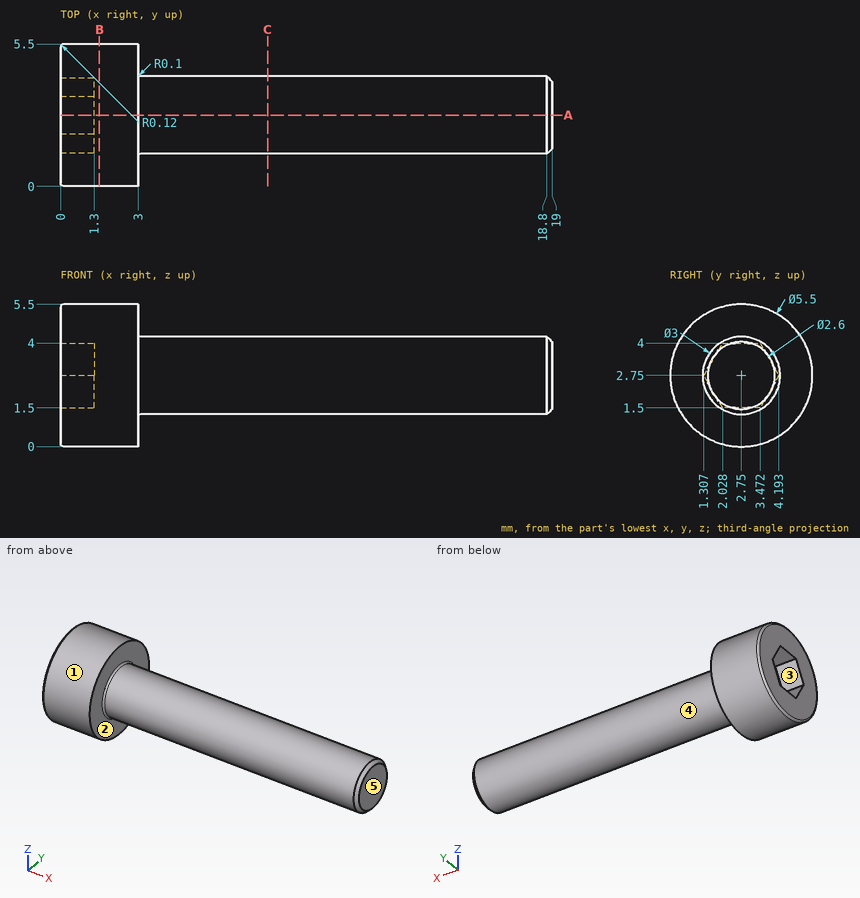
Verification items for this drawing (mm, ordinates from the low corner). A direction names the side the tool comes from. Give positions to 0.01 mm unless a question says otherwise; leave off trailing zeros. Loops run counter-clockwise (first coordinate to the right, second up) from the corner with the lowest first, then second, coordinate; pieces in that order, holes last. Notation, with made-up numbers: (11, -25.75) - (58, -25.75) arc R10 ccw to (58, -9.75) - close; hole circle Ø5 at (37, 29). An arc over 180 degrees is marked (long way). Write item = value, one per line. Start each with the question number.
Q1. Mould release check, pull along Z, two halves, no side actions. Record for the marked faces 1, 2 and 3: released by +Z, released by -Z, zero draft, split by the parting line, or undercut.
Q2. Tool access check on the marked faces 4 and 5. Record the directions out of +Z, -Z, +X, -X, +Y, -Y that give a thin tool (end or side, any length) a straight path to the whole face; none if there is none.
Q3. Cross-section at A-A, the plane y = 2.75. Enter the section's corners in (x, z).
Q4. Cross-section at B-B, the plane x = 1.5. Enter the section's corners in (y, z).
Q5. Cross-section at C-C, the plane x = 8. Enter the section's corners in (y, z).
Q6. Thickness scan on line 1 (X direction, y = 0.6, z = 2.4); line 2 (X direction, y = 3.4, z = 2.35); line 3 (Z direction, x = 17.75, y = 2). Record the ranges inside material, lowest first.
Q7. Depth check by flat-ended pin: P1, Ø3, axis at y = 1.5, z = 2.5, coming from the -X side; P2, Ø1.2, axis at y = 2.5, z = 3, coming from the -X side. Enter the tip coordinate at first touch or a pass-through.
Answer key:
q1.face_1 = split by the parting line
q1.face_2 = zero draft
q1.face_3 = undercut
q2.face_4 = +X
q2.face_5 = +Z, -Z, +X, +Y, -Y
q3.outline = (0, 0.12) arc R0.12 ccw to (0.12, 0) - (3, 0) - (3, 1.15) arc R0.1 cw to (3.1, 1.25) - (18.8, 1.25) - (19, 1.45) - (19, 4.05) - (18.8, 4.25) - (3.1, 4.25) arc R0.1 cw to (3, 4.35) - (3, 5.5) - (0.12, 5.5) arc R0.12 ccw to (0, 5.38) - (0, 4) - (1.3, 4) - (1.3, 1.5) - (0, 1.5) - close
q4.outline = circle Ø5.5 at (2.75, 2.75)
q5.outline = circle Ø3 at (2.75, 2.75)
q6.line_1 = 0 to 3
q6.line_2 = 1.3 to 19
q6.line_3 = 1.45 to 4.05
q7.P1 = 0
q7.P2 = 1.3
